Geometry check sheet. Reference: the model listing, model coordinates, mm. A direction names the side the tool comes from. Round coordinates to 2 decimals unless told otherwise and drop trailing zeros. Write each loop counter-clockwise with the first axis right and the second up, starting at its lowest first coordinate (ties: lowest second). Pieces come first, ordered by that corner, then holes. Notation, with made-up numbers: (-33, 12.5) -> (-8, 12.5) arc R14 ccw to (-8, 38.5) -> close; hole circle Ø4 at (-8.5, 22.5). An arc over 180 degrees is marked (long way). Use a Markdown table: item, result.
```python
from build123d import *

# Parameters (mm, degrees)
SKETCH2_R           = 14.213072664
BOSS_EXTRUDE2_DEPTH = 24
SKETCH4_R           = 15
BOSS_EXTRUDE4_DEPTH = 25
FILLET2_R           = 20


with BuildPart() as part:
    # Sketch2 → Boss-Extrude2 (new body)
    with BuildSketch(Plane(origin=(0, 0, 0), x_dir=(1, 0, 0), z_dir=(0, 1, 0))):
        with BuildLine():
            Line((0, 0), (0, 75.803054209))
            Line((0, 75.803054209), (123.17996309, 75.803054209))
            ThreePointArc((123.17996309, 75.803054209), (161.081490195, 37.901527105), (123.17996309, 0))
            Line((123.17996309, 0), (0, 0))
        make_face()
        with Locations(Location((123.17996309, 37.901527105, 0), (0, 0, 270))):
            Circle(SKETCH2_R, mode=Mode.SUBTRACT)
    extrude(amount=BOSS_EXTRUDE2_DEPTH)

    # Sketch4 → Boss-Extrude4 (add)
    with BuildSketch(Plane.XY):
        with BuildLine():
            Line((0, 60), (0, 24))
            Line((0, 24), (79.971353362, 24))
            Line((79.971353362, 24), (79.971353362, 58.486424634))
            ThreePointArc((79.971353362, 58.486424634), (40.756923216, 99.992837699), (0, 60))
        make_face()
        with Locations((40, 60)):
            Circle(SKETCH4_R, mode=Mode.SUBTRACT)
    extrude(amount=-BOSS_EXTRUDE4_DEPTH)

    # Fillet2
    fillet2_edges = [part.edges().sort_by_distance(p)[0] for p in [
        (0, 12, -75.803054209),
    ]]
    fillet(fillet2_edges, radius=FILLET2_R)


solid = part.part
```
(1) Section check A-A on x = 40. Record the cut outline in (y, z), plus the area to 3 significant figures.
A:
| item | result |
|---|---|
| outline | (0, -75.8) -> (24, -75.8) -> (24, -25) -> (45, -25) -> (45, 0) -> (0, 0) -> close; (75, -25) -> (100, -25) -> (100, 0) -> (75, 0) -> close |
| area | 2,970 mm2 |
(2) Section check C-C on z = -19. Record the cut outline in (x, y), plus the area to 3 significant figures.
A:
| item | result |
|---|---|
| outline | (0, 0) -> (156.03, 0) -> (156.03, 24) -> (79.97, 24) -> (79.97, 58.49) arc R40 ccw (long way) to (0, 60) -> close; hole circle Ø30 at (40, 60) |
| area | 8,430 mm2 |
(3) Section check D-D on z = -42.5. Record the cut outline in (x, y), plus the area to 3 significant figures.
A:
| item | result |
|---|---|
| outline | (0, 0) -> (109.73, 0) -> (109.73, 24) -> (0, 24) -> close; (136.63, 0) -> (160.8, 0) -> (160.8, 24) -> (136.63, 24) -> close |
| area | 3,210 mm2 |
(4) Section check B-B on y = 65. Record the cut outline in (x, z), plus the area to 3 significant figures.
A:
| item | result |
|---|---|
| outline | (0.31, -25) -> (25.86, -25) -> (25.86, 0) -> (0.31, 0) -> close; (54.14, -25) -> (79.69, -25) -> (79.69, 0) -> (54.14, 0) -> close |
| area | 1,280 mm2 |
(5) Release check for a two-part mould opening along X. For faces 1 (the face through (0, 24, -21)), 2 (the face through (28, 51, -12)), 3 (the face through (41.647, 99.966, -12.325)), 4 (the face through (82, 24, -47)) record: +X half, -X half, draft (parallel to the pull), parting line (faces both ways), or undercut.
A:
| item | result |
|---|---|
| face 1 | -X half |
| face 2 | undercut |
| face 3 | parting line |
| face 4 | draft |
(6) Thickness scan on line 1 (X direction, y = 59, z = -23); line 2 (Y direction, x = 141, z = -52); line 3 (Z direction, x = 57.5, y = 39). Record the ranges inside material, lowest first.
A:
| item | result |
|---|---|
| line 1 | x = 0 to 25.03, 54.97 to 79.99 |
| line 2 | y = 0 to 24 |
| line 3 | z = -25 to 0 |
(7) Access from +Z, -Z, +X, -X, +Y, -Y to the whole of each face (thin tool, end or side, straight path). Record for faces 5 (the face through (5.703, 12.168, -69.789)), 6 (the face through (31, 46, -25)).
A:
| item | result |
|---|---|
| face 5 | -Z, -X, +Y, -Y |
| face 6 | -Z, +X, -X, +Y |
(8) Gauge pin test, flat ends, axial feed: pin 1 Ø7.5 at (y, z) = (38.5, -11.5) entering from +X; pin 2 Ø2 at (x, y) = (58, 29) entering from -Z; pin 3 Ø2 at (x, z) = (25.5, -35.5) entering from +Y; pin 4 Ø10 at (x, z) = (119, -9) entering from -Y. Record the tip position at first contact, or that the pin passes through.
A:
| item | result |
|---|---|
| pin 1 | stops at x = 79.97 |
| pin 2 | stops at z = -25 |
| pin 3 | stops at y = 24 |
| pin 4 | stops at y = 0 |
